Read the model definition and answer for the solid it produces. Units are mm, in the model's axes. Face numbers are marked on the shaded views. A direction names the side the tool comes from. Coordinates: 2 decimals unless noted, no trailing zeros. Loops run counter-clockwise (first coordinate to the right, second up) from the corner with the lowest first, then second, coordinate; pieces in that order, holes last. Notation, with made-up numbers: M 69.5,14 L 81.5,14 A20 ccw 81.5,41 Z; hole C 54.5,18 d8. An arc over 180 degrees is marked long. Use one line per item in the form item = value. Start each with the question number.
1. For a pull along Y with two mould halves and no side action, classify the marked faces 1, 2 and 3 as released by +Y, released by -Y, zero draft, split by the parting line, or undercut.
2. The part is cut by section D-D (y = -2.25). Give the vertices of the cut face in (x, z), plus the area to 3 significant figures.
3. The part is cut by section B-B (x = 3.15). Give the vertices of the cut face in (y, z).
4. Flat-ended cylindrical pins translate along their axes: pin 1 (1 mm diameter, centred on x = 4.5, y = -2, fed in from -Z); pin 2 (1.8 mm diameter, centred on y = -2.5, z = 1, fed in from -X); pin 3 (0.6 mm diameter, centred on x = 6.5, z = -0.5, fed in from -Y); pin 4 (3 mm diameter, centred on y = -3.5, z = -0.5, fed in from -X). Find the tip coordinate at first contact, or state that the pin passes through.
5. A tool of negligible diameter and unlimited length cuts with its end or side. For the marked faces 4, 5, 6, 7 and 8, from which of +Z, -Z, +X, -X, +Y, -Y can it reach the whole face along a straight path? Write none if from no direction.
6. Find the intervals of material crossed by probe 1 along Z at (x, y) = (2, -0.4); probe 2 along X at (y, z) = (-0.25, 2); probe 3 along Z at (x, y) = (3, -0.95), in increasing order. Write a range as [from, to].
7. The part is cut by section C-C (z = 2). Give the vertices of the cut face in (x, y), plus the area to 3 significant figures.
8. The part is cut by section A-A (z = -0.25). Give the vertices of the cut face in (x, y), plus the area to 3 significant figures.
from build123d import *

# Parameters (mm, degrees)
SKETCH001_W  = 6
SKETCH001_H  = 6
PAD001_DEPTH = 0.1
FILLET001_R  = 0.3
PAD008_DEPTH = 0.7
FILLET003_R  = 0.29
PAD009_DEPTH = 0.7
FILLET004_R  = 0.29
PAD010_DEPTH = 0.7
FILLET005_R  = 0.29
SKETCH_W     = 6
SKETCH_H     = 6
PAD_DEPTH    = 3.5
FILLET_R     = 0.3
SKETCH004_R  = 0.5
PAD003_DEPTH = 0.6
SKETCH003_R  = 0.5
PAD004_DEPTH = 0.6
SKETCH005_R  = 0.5
PAD002_DEPTH = 0.6
SKETCH002_R  = 0.5
PAD005_DEPTH = 0.6
SKETCH006_R  = 1.75
PAD006_DEPTH = 3.8
FILLET006_R  = 0.1
PAD007_DEPTH = 0.7
FILLET002_R  = 0.29


with BuildPart() as fillet001:
    # Sketch001 → Pad001 (new body)
    with BuildSketch(Plane.XY.offset(3.5)):
        with Locations((3.15, -2.25)):
            Rectangle(SKETCH001_W, SKETCH001_H)
    extrude(amount=PAD001_DEPTH)

    # Fillet001
    fillet001_edges = [fillet001.edges().sort_by_distance(p)[0] for p in [
        (6.15, -5.25, 3.55),
        (0.15, -5.25, 3.55),
        (6.15, 0.75, 3.55),
        (0.15, 0.75, 3.55),
    ]]
    fillet(fillet001_edges, radius=FILLET001_R)


with BuildPart() as fillet003:
    # Sketch008 → Pad008 (new body)
    with BuildSketch(Plane.XZ.offset(0.35)):
        Polygon((-0.15, 1.5), (0.15, 1.5), (0.15, -0.5), (-0.15, -1.5), (0.15, -2.5), (0.15, -3.5), (-0.15, -3.5), (-0.15, -2.5), (-0.45, -1.5), (-0.15, -0.5), align=None)
    extrude(amount=-PAD008_DEPTH)

    # Fillet003
    fillet003_edges = [fillet003.edges().sort_by_distance(p)[0] for p in [
        (-0.15, 0, -2.5),
        (-0.15, 0, -0.5),
        (-0.45, 0, -1.5),
        (-0.15, 0, 1.5),
        (0.15, 0, -0.5),
        (-0.15, 0, -1.5),
        (0.15, 0, -2.5),
    ]]
    fillet(fillet003_edges, radius=FILLET003_R)


with BuildPart() as fillet004:
    # Sketch009 → Pad009 (new body)
    with BuildSketch(Plane.XZ.offset(4.85)):
        Polygon((6.45, 1.5), (6.15, 1.5), (6.15, -0.5), (6.45, -1.5), (6.15, -2.5), (6.15, -3.5), (6.45, -3.5), (6.45, -2.5), (6.75, -1.5), (6.45, -0.5), align=None)
    extrude(amount=-PAD009_DEPTH)

    # Fillet004
    fillet004_edges = [fillet004.edges().sort_by_distance(p)[0] for p in [
        (6.45, -4.5, -2.5),
        (6.45, -4.5, -0.5),
        (6.75, -4.5, -1.5),
        (6.45, -4.5, 1.5),
        (6.15, -4.5, -0.5),
        (6.45, -4.5, -1.5),
        (6.15, -4.5, -2.5),
    ]]
    fillet(fillet004_edges, radius=FILLET004_R)


with BuildPart() as fillet005:
    # Sketch010 → Pad010 (new body)
    with BuildSketch(Plane.XZ.offset(0.35)):
        Polygon((6.45, 1.5), (6.15, 1.5), (6.15, -0.5), (6.45, -1.5), (6.15, -2.5), (6.15, -3.5), (6.45, -3.5), (6.45, -2.5), (6.75, -1.5), (6.45, -0.5), align=None)
    extrude(amount=-PAD010_DEPTH)

    # Fillet005
    fillet005_edges = [fillet005.edges().sort_by_distance(p)[0] for p in [
        (6.45, 0, -2.5),
        (6.45, 0, -0.5),
        (6.75, 0, -1.5),
        (6.45, 0, 1.5),
        (6.15, 0, -0.5),
        (6.45, 0, -1.5),
        (6.15, 0, -2.5),
    ]]
    fillet(fillet005_edges, radius=FILLET005_R)


with BuildPart() as fillet_body:
    # Sketch → Pad (new body)
    with BuildSketch(Plane.XY):
        with Locations((3.15, -2.25)):
            Rectangle(SKETCH_W, SKETCH_H)
    extrude(amount=PAD_DEPTH)

    # Fillet
    fillet_edges = [fillet_body.edges().sort_by_distance(p)[0] for p in [
        (6.15, 0.75, 1.75),
        (6.15, -5.25, 1.75),
        (0.15, -5.25, 1.75),
        (0.15, 0.75, 1.75),
    ]]
    fillet(fillet_edges, radius=FILLET_R)


with BuildPart() as pad003:
    # Pad003 base: copy of Fillet body
    add(fillet_body.part)

    # Sketch004 → Pad003 (new body)
    with BuildSketch(Plane.XY.offset(3.5)):
        with Locations((5.15, -0.25)):
            Circle(SKETCH004_R)
    extrude(amount=PAD003_DEPTH)


with BuildPart() as pad004:
    # Pad004 base: copy of Fillet body
    add(fillet_body.part)

    # Sketch003 → Pad004 (new body)
    with BuildSketch(Plane.XY.offset(3.5)):
        with Locations((5.15, -4.25)):
            Circle(SKETCH003_R)
    extrude(amount=PAD004_DEPTH)


with BuildPart() as pad002:
    # Pad002 base: copy of Fillet body
    add(fillet_body.part)

    # Sketch005 → Pad002 (new body)
    with BuildSketch(Plane.XY.offset(3.5)):
        with Locations((1.15, -0.25)):
            Circle(SKETCH005_R)
    extrude(amount=PAD002_DEPTH)


with BuildPart() as pad005:
    # Pad005 base: copy of Fillet body
    add(fillet_body.part)

    # Sketch002 → Pad005 (new body)
    with BuildSketch(Plane.XY.offset(3.5)):
        with Locations((1.15, -4.25)):
            Circle(SKETCH002_R)
    extrude(amount=PAD005_DEPTH)


with BuildPart() as fillet006:
    # Pad006 base: copy of Fillet body
    add(fillet_body.part)

    # Sketch006 → Pad006 (new body)
    with BuildSketch(Plane.XY.offset(3.5)):
        with Locations((3.15, -2.25)):
            Circle(SKETCH006_R)
    extrude(amount=PAD006_DEPTH)

    # Fillet006
    fillet006_edges = [fillet006.edges().sort_by_distance(p)[0] for p in [
        (1.4, -2.25, 7.3),
    ]]
    fillet(fillet006_edges, radius=FILLET006_R)


with BuildPart() as obj1:
    # Sketch007 → Pad007 (new body)
    with BuildSketch(Plane.XZ.offset(4.85)):
        Polygon((-0.15, 1.5), (0.15, 1.5), (0.15, -0.5), (-0.15, -1.5), (0.15, -2.5), (0.15, -3.5), (-0.15, -3.5), (-0.15, -2.5), (-0.45, -1.5), (-0.15, -0.5), align=None)
    extrude(amount=-PAD007_DEPTH)

    # Fillet002
    fillet002_edges = [obj1.edges().sort_by_distance(p)[0] for p in [
        (-0.15, -4.5, -2.5),
        (-0.15, -4.5, -0.5),
        (-0.45, -4.5, -1.5),
        (-0.15, -4.5, 1.5),
        (0.15, -4.5, -0.5),
        (-0.15, -4.5, -1.5),
        (0.15, -4.5, -2.5),
    ]]
    fillet(fillet002_edges, radius=FILLET002_R)

    add(fillet001.part)
    add(fillet003.part)
    add(fillet004.part)
    add(fillet005.part)
    add(pad003.part)
    add(pad004.part)
    add(pad002.part)
    add(pad005.part)
    add(fillet006.part)


solid = obj1.part
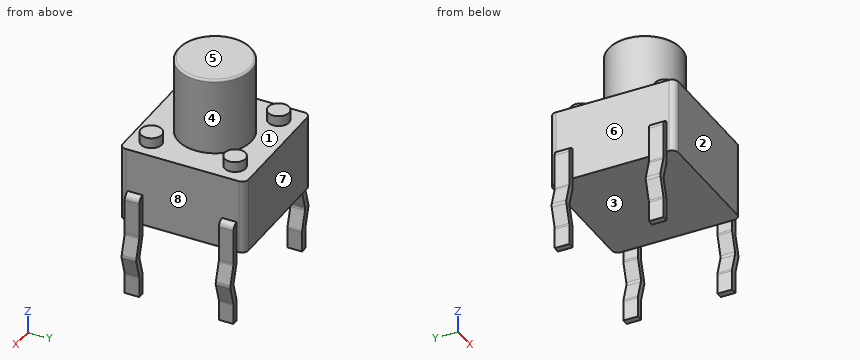
Computed values:
q1.face_1 = undercut
q1.face_2 = released by -Y
q1.face_3 = zero draft
q2.outline = M 0.15,0 L 6.15,0 L 6.15,3.6 L 4.9,3.6 L 4.9,7.2 A0.1 ccw 4.8,7.3 L 1.5,7.3 A0.1 ccw 1.4,7.2 L 1.4,3.6 L 0.15,3.6 Z
q2.area = 34.5 mm²
q3.outline = M -5.25,0 L 0.75,0 L 0.75,3.6 L -0.5,3.6 L -0.5,7.2 A0.1 ccw -0.6,7.3 L -3.9,7.3 A0.1 ccw -4,7.2 L -4,3.6 L -5.25,3.6 Z
q4.pin_1 = 0
q4.pin_2 = 0.15
q4.pin_3 = -4.85
q4.pin_4 = -0.44
q5.face_4 = +Z
q5.face_5 = +Z, +X, -X, +Y, -Y
q5.face_6 = +Z, -X
q5.face_7 = +Z, -Z, +X, -X, +Y
q5.face_8 = +Z, +X
q6.probe_1 = [0, 3.6]
q6.probe_2 = [0.15, 6.15]
q6.probe_3 = [0, 7.3]
q7.outline = M 0.15,-4.95 A0.3 ccw 0.45,-5.25 L 5.85,-5.25 A0.3 ccw 6.15,-4.95 L 6.15,0.45 A0.3 ccw 5.85,0.75 L 0.45,0.75 A0.3 ccw 0.15,0.45 Z
q7.area = 35.9 mm²
q8.outline = M -0.15,-4.85 L 0.15,-4.85 L 0.15,-4.15 L -0.15,-4.15 Z; M -0.15,-0.35 L 0.15,-0.35 L 0.15,0.35 L -0.15,0.35 Z; M 6.15,-4.85 L 6.45,-4.85 L 6.45,-4.15 L 6.15,-4.15 Z; M 6.15,-0.35 L 6.45,-0.35 L 6.45,0.35 L 6.15,0.35 Z
q8.area = 0.840 mm²
